Part model, mm, in its own coordinate system. A direction names the side the tool comes from. Round coordinates to 2 decimals unless told otherwise and drop trailing zeros. Write each loop counter-clockwise with the first axis right and the second up, starting at its lowest first coordinate (ties: lowest second). Pieces come first, ordered by that corner, then holes. Notation, with made-up numbers: (74.5, -8.75) -> (113.5, -8.75) arc R18 cw to (113.5, -4.75) -> close; hole circle Ø8 at (42.25, 86.25). An arc over 180 degrees is marked (long way). Return JSON: item names as keys, results as strings. Group by question number.
```python
from build123d import *

# Parameters (mm, degrees)
BASE_FLANGE1_DEPTH = 72
FILLET1_R          = 5
SKETCH6_R          = 2.1
CUT_EXTRUDE1_DEPTH = 74.524009684
SKETCH7_R          = 2.1
CUT_EXTRUDE2_DEPTH = 74.524009684
LPATTERN1_COUNT    = 9
LPATTERN1_PITCH    = 8


# Sheet-metal steps are written as plain solids
with BuildPart() as part:
    # Sketch1 → Base-Flange1 (new body)
    with BuildSketch(Plane(origin=(0, 0, 0), x_dir=(0, 0, -1), z_dir=(1, 0, 0))):
        with BuildLine():
            Line((0, 11.3), (0, 2.6))
            ThreePointArc((0, 2.6), (-0.761522369, 0.761522369), (-2.6, 0))
            Line((-2.6, 0), (-11.3, 0))
            Line((-11.3, 0), (-11.3, 1.6))
            Line((-11.3, 1.6), (-2.6, 1.6))
            ThreePointArc((-2.6, 1.6), (-1.892893219, 1.892893219), (-1.6, 2.6))
            Line((-1.6, 2.6), (-1.6, 11.3))
            Line((-1.6, 11.3), (0, 11.3))
        make_face()
    extrude(amount=BASE_FLANGE1_DEPTH)

    # Fillet1
    fillet1_edges = [part.edges().sort_by_distance(p)[0] for p in [
        (72, 11.3, 0.8),
        (72, 0.8, 11.3),
        (0, 11.3, 0.8),
        (0, 0.8, 11.3),
    ]]
    fillet(fillet1_edges, radius=FILLET1_R)

    # Sketch6 → Cut-Extrude1 (cut, through all)
    with BuildSketch(Plane.XY.offset(1.6)):
        with Locations((4, 6.5)):
            Circle(SKETCH6_R)
    cut_extrude1 = extrude(amount=-CUT_EXTRUDE1_DEPTH, mode=Mode.SUBTRACT)

    # Sketch7 → Cut-Extrude2 (cut, through all)
    with BuildSketch(Plane(origin=(0, 1.6, 0), x_dir=(1, 0, 0), z_dir=(0, 1, 0))):
        with Locations(Location((4, -6.5, 0), (0, 0, 270))):
            Circle(SKETCH7_R)
    cut_extrude2 = extrude(amount=-CUT_EXTRUDE2_DEPTH, mode=Mode.SUBTRACT)

    # LPattern1: Cut-Extrude1, Cut-Extrude2 ×9
    with Locations(*[(i * LPATTERN1_PITCH, 0, 0) for i in range(1, LPATTERN1_COUNT)]):
        add(cut_extrude1, mode=Mode.SUBTRACT)
        add(cut_extrude2, mode=Mode.SUBTRACT)


solid = part.part
```
Item 1: Cut at B-B (y = 1). State how many separate pieces and enclosed holes the cut face has, then the cut area to 3 significant figures.
Item 2: Which spindle directions (+Z, -Z, +X, -X, +Y, -Y) get a long thin tool onto all of the face, cutting with end or side? Do faces 1 (the face through (35, 9, 1.6)), 2 (the face through (1.5, 0.81, 9.87)). Say none if no direction does.
Item 3: Cut at C-C (x = 7). Write the cut outline in (y, z), then the cut area to 3 significant figures.
Item 4: Flat gauge pins, fed straight in: P1, Ø1.5, axis at x = 29, y = 1, coming from the -Z side; P2, Ø2.5, axis at x = 52, y = 6.5, coming from the -Z side; P3, Ø1.5, axis at x = 17.5, y = 3.5, coming from the +Z side; P4, Ø5.5, axis at x = 44, z = 6.5, coming from the +Y side. Where does each tip first touch, or does it go through?
Item 5: Wall check: L1, parallel to Y at x = 47, z = 9.75; L2, parallel to Z at x = 68.5, y = 1.5; L3, parallel to Y at x = 28, z = 1. Give the ranges that are in metal, low to high.
Item 6: Two-plate mould, pull along Y, no slides. Class faces 3 (the face through (1.5, 9.87, 0.79)), 4 (the face through (69.13, 8.27, 0.81)), 5 (the face through (33.95, 0.81, 6.04)), 6 (the face through (43.727, 8.582, 0.811)): released by +Y, released by -Y, zero draft, split by the parting line, or undercut.
Item 7: Cut at A-A (x = 36). Write the cut outline in (y, z), then the cut area to 3 significant figures.
Checks:
{
 "1": {"separate pieces": "1", "enclosed holes": "9", "area": "639 mm2"},
 "2": {"face 1": "+Z, +X, -X, +Y", "face 2": "+Z, -X, +Y, -Y"},
 "3": {"outline": "(0, 2.6) arc R2.6 ccw to (2.6, 0) -> (11.3, 0) -> (11.3, 1.6) -> (2.6, 1.6) arc R1 cw to (1.6, 2.6) -> (1.6, 11.3) -> (0, 11.3) -> close", "area": "32.4 mm2"},
 "4": {"P1": "stops at z = 0.14", "P2": "passes through", "P3": "stops at z = 1.6", "P4": "stops at y = 1.6"},
 "5": {"L1": "y = 0 to 1.6", "L2": "z = 0.24 to 4.46, 8.54 to 11.07", "L3": "y = 0.55 to 4.4, 8.6 to 11.3"},
 "6": {"face 3": "released by +Y", "face 4": "undercut", "face 5": "zero draft", "face 6": "undercut"},
 "7": {"outline": "(0, 2.6) arc R2.6 ccw to (2.6, 0) -> (4.4, 0) -> (4.4, 1.6) -> (2.6, 1.6) arc R1 cw to (1.6, 2.6) -> (1.6, 4.4) -> (0, 4.4) -> close; (0, 8.6) -> (1.6, 8.6) -> (1.6, 11.3) -> (0, 11.3) -> close; (8.6, 0) -> (11.3, 0) -> (11.3, 1.6) -> (8.6, 1.6) -> close", "area": "18.9 mm2"}
}
